from build123d import *

# Parameters (mm, degrees)
BOSS_EXTRUDE1_DEPTH = 4
SKETCH2_W           = 92.5
SKETCH2_H           = 8
CUT_EXTRUDE1_DEPTH  = 187.792378648
SKETCH3_R           = 1.25
CUT_EXTRUDE2_DEPTH  = 187.792378648
SKETCH4_R           = 3.25
CUT_EXTRUDE3_DEPTH  = 187.792378648
FILLET1_R           = 10
FILLET2_R           = 5
CUT_EXTRUDE4_DEPTH  = 187.792378648


with BuildPart() as part:
    # Sketch1 → Boss-Extrude1 (new body)
    with BuildSketch(Plane(origin=(0, 0, 0), x_dir=(1, 0, 0), z_dir=(0, 1, 0))):
        Polygon((155.594010768, -30), (63.094010768, -30), (63.094010768, -50), (78.094010768, -75.980762114), (86.754264805, -70.980762114), (74.641016151, -50), (163.094010768, -50), (170.594010768, -30), (170.594010768, 30), (155.594010768, 30), align=None)
    extrude(amount=BOSS_EXTRUDE1_DEPTH)

    # Sketch2 → Cut-Extrude1 (cut, through all)
    with BuildSketch(Plane(origin=(0, 0, 0), x_dir=(1, 0, 0), z_dir=(0, 1, 0))):
        with Locations((109.344010768, -34)):
            Rectangle(SKETCH2_W, SKETCH2_H)
    extrude(amount=CUT_EXTRUDE1_DEPTH, mode=Mode.SUBTRACT)

    # Sketch3 → Cut-Extrude2 (cut, through all)
    with BuildSketch(Plane(origin=(0, 4, 0), x_dir=(1, 0, 0), z_dir=(0, 1, 0))):
        with Locations(Location((75.174137787, -60.923393759, 0), (0, 0, 270))):
            Circle(SKETCH3_R)
        with Locations(Location((79.924137787, -69.150635095, 0), (0, 0, 270))):
            Circle(SKETCH3_R)
    extrude(amount=-CUT_EXTRUDE2_DEPTH, mode=Mode.SUBTRACT)

    # Sketch4 → Cut-Extrude3 (cut, through all)
    with BuildSketch(Plane(origin=(0, 4, 0), x_dir=(1, 0, 0), z_dir=(0, 1, 0))):
        with Locations(Location((163.094010768, 15, 0), (0, 0, 270))):
            Circle(SKETCH4_R)
        with Locations(Location((163.094010768, -15, 0), (0, 0, 270))):
            Circle(SKETCH4_R)
    extrude(amount=-CUT_EXTRUDE3_DEPTH, mode=Mode.SUBTRACT)

    # Fillet1
    # the kernel refuses this fillet: 10 mm, written as the material it takes off along each edge
    with BuildSketch(Plane(origin=(63.094010768, -6.698729811, 50), x_dir=(0, 0, -1), z_dir=(0, 1, 0))) as fillet1_piece_1:
        with BuildLine():
            CenterArc((FILLET1_R * 0.267949192431, -FILLET1_R), FILLET1_R, 90, 30)
            Line((-FILLET1_R * 0.232050807569, -FILLET1_R * 0.133974596216), (0, 0))
            Line((0, 0), (FILLET1_R * 0.267949192431, 0))
        make_face()
    extrude(amount=17.397459622, mode=Mode.SUBTRACT)
    with BuildSketch(Plane(origin=(63.094010768, -25, 38), x_dir=(1, 0, 0), z_dir=(0, 1, 0))) as fillet1_piece_2:
        with BuildLine():
            CenterArc((FILLET1_R, -FILLET1_R), FILLET1_R, 90, 90)
            Line((0, -FILLET1_R), (0, 0))
            Line((0, 0), (FILLET1_R, 0))
        make_face()
    extrude(amount=54, mode=Mode.SUBTRACT)
    with BuildSketch(Plane(origin=(163.094010768, -17.325011704, 50), x_dir=(0.35112344158838954, 0, -0.9363291775690453), z_dir=(0, 1, 0))) as fillet1_piece_3:
        with BuildLine():
            CenterArc((FILLET1_R * 0.693000468165, FILLET1_R), FILLET1_R, 200.55604522, 69.44395478)
            Line((-FILLET1_R * 0.243328709404, FILLET1_R * 0.648876558412), (0, 0))
            Line((0, 0), (FILLET1_R * 0.693000468165, 0))
        make_face()
    extrude(amount=38.650023408, mode=Mode.SUBTRACT)
    with BuildSketch(Plane(origin=(170.594010768, -4.533364544, 30), x_dir=(0, 0, -1), z_dir=(0, 1, 0))) as fillet1_piece_4:
        with BuildLine():
            CenterArc((FILLET1_R * 0.181334581773, FILLET1_R), FILLET1_R, 249.44395478, 20.55604522)
            Line((-FILLET1_R * 0.169788859816, FILLET1_R * 0.063670822431), (0, 0))
            Line((0, 0), (FILLET1_R * 0.181334581773, 0))
        make_face()
    extrude(amount=13.066729089, mode=Mode.SUBTRACT)

    # Fillet2
    fillet2_edges = [part.edges().sort_by_distance(p)[0] for p in [
        (74.641016151, 2, 50),
    ]]
    fillet(fillet2_edges, radius=FILLET2_R)

    # Sketch5 → Cut-Extrude4 (cut, through all)
    with BuildSketch(Plane(origin=(0, 4, 0), x_dir=(1, 0, 0), z_dir=(0, 1, 0))):
        with BuildLine():
            ThreePointArc((83.16294466, -68.116547777), (80.630175188, -70.185907233), (77.592361621, -71.397871955))
            ThreePointArc((77.592361621, -71.397871955), (76.093210222, -70.461098192), (77.029983985, -68.961946793))
            ThreePointArc((77.029983985, -68.961946793), (79.361329281, -68.031834332), (81.305082597, -66.443721261))
            ThreePointArc((81.305082597, -66.443721261), (83.070426886, -66.351203487), (83.16294466, -68.116547777))
        make_face()
    extrude(amount=-CUT_EXTRUDE4_DEPTH, mode=Mode.SUBTRACT)


solid = part.part
Verification items for the finished model (mm, model axes). A direction names the side the tool comes from. Round coordinates to 2 decimals unless told otherwise and drop trailing zeros. Loops run counter-clockwise (first coordinate to the right, second up) from the corner with the lowest first, then second, coordinate; pieces in that order, holes last. Notation, with made-up numbers: (43.25, 44) - (50.25, 44) arc R16 ccw to (50.25, 61) - close; hole circle Ø4 at (33.25, -11). An arc over 180 degrees is marked (long way). Answer in a Markdown table with one row per item. Add a question column.
Q1. Material ranges on line 1 (X direction, y = 1.15, z = -15); line 2 (Z direction, x = 83, y = 0.4); line 3 (Z direction, x = 124.5, y = 2.35), recorded low to high.
Q2. Tool access check on faces 5 (the face through (155.594, 2, 4)), 6 (the face through (79.33, 2.03, 68.05)), 7 (the face through (82.917, 1.972, 64.335)). Record the directions out of +Z, -Z, +X, -X, +Y, -Y that give a thin tool (end or side, any length) a straight path to the whole face; none if there is none.
Q3. Section check D-D on x = 150.5. Enter the section's corners in (y, z), plus the area to 3 significant figures.
Q4. Section check C-C on z = -3. Enter the section's corners in (x, y), plus the area to 3 significant figures.
Q5. Section check B-B on y = 0.9. Enter the section's corners in (x, z).
Q6. Gauge pin test, flat ends, axial feed: pin 1 (2 mm diameter, centred on x = 75.17, z = 60.92, fed in from -Y); pin 2 (2 mm diameter, centred on x = 118.5, y = 1, fed in from +Z); pin 3 (2 mm diameter, centred on x = 131.5, y = 1.5, fed in from -Z); pin 4 (1.5 mm diameter, centred on y = 0.5, z = 56, fed in from +X). Record the tip position at first contact, or that the pin passes through.
Q7. Section check A-A on z = 15. Enter the section's corners in (x, y), plus the area to 3 significant figures.
Q8. Release check for a two-part mould opening along X. For faces 1 (the face through (160, 2, 14)), 2 (the face through (114, 2, 38)), 3 (the face through (71.17, 1.97, 63.99)), 4 (the face through (76.1, 2.03, 70.49)) record: pulls with the +X half, pulls with the -X half, needs draft (parallel to the pull), parting line crosses it, or undercut.
Found:
| question | item | result |
|---|---|---|
| 1 | line 1 | x = 155.59 to 159.84, 166.34 to 170.59 |
| 1 | line 2 | z = 38 to 50.01, 64.48 to 66.29, 68.29 to 73.15 |
| 1 | line 3 | z = 38 to 50 |
| 2 | face 5 | -Z, -X, +Y, -Y |
| 2 | face 6 | +Y, -Y |
| 2 | face 7 | +X, +Y, -Y |
| 3 | outline | (0, 38) - (4, 38) - (4, 50) - (0, 50) - close |
| 3 | area | 48.0 mm² |
| 4 | outline | (155.59, 0) - (170.59, 0) - (170.59, 4) - (155.59, 4) - close |
| 4 | area | 60.0 mm² |
| 5 | outline | (63.1, 47.66) arc R10 ccw to (73.09, 38) - (155.59, 38) - (155.59, -30) - (170.59, -30) - (170.59, 28.19) arc R10 ccw to (169.96, 31.7) - (165.53, 43.51) arc R10 ccw to (156.16, 50) - (83.3, 50) arc R5 cw to (78.97, 57.5) - (86.75, 70.98) - (78.09, 75.98) - (64.43, 52.32) arc R10 ccw to start; hole circle Ø2.5 at (75.17, 60.92); hole (77.03, 68.96) arc R8.25 cw to (81.31, 66.44) arc R1.25 ccw to (83.16, 68.12) arc R10.75 ccw to (77.59, 71.4) arc R1.25 ccw to start; hole circle Ø6.5 at (163.09, -15); hole circle Ø6.5 at (163.09, 15) |
| 6 | pin 1 | passes through |
| 6 | pin 2 | stops at z = 50 |
| 6 | pin 3 | stops at z = 38 |
| 6 | pin 4 | stops at x = 78.62 |
| 7 | outline | (155.59, 0) - (159.84, 0) - (159.84, 4) - (155.59, 4) - close; (166.34, 0) - (170.59, 0) - (170.59, 4) - (166.34, 4) - close |
| 7 | area | 34.0 mm² |
| 8 | face 1 | undercut |
| 8 | face 2 | needs draft |
| 8 | face 3 | pulls with the -X half |
| 8 | face 4 | undercut |
